Work out the finished part from the listing and answer in its coordinate system (mm). A direction names the side the tool comes from. Give positions to 0.01 mm unless a question says otherwise; leave off trailing zeros. Write each loop counter-clockwise with the first axis right and the second up, starting at its lowest first coordinate (ties: lowest second). Pieces come first, ordered by that corner, then holes.
1) Determine the mould class of faces 1 (the face through (-25, 6, -50)), 2 (the face through (-50, 1, -25)), 3 (the face through (-2.175, 0.789, -46.036)) for opening direction X: pulls with the +X half, pulls with the -X half, needs draft (parallel to the pull), parting line crosses it, or undercut.
2) Find section D-D (z = -28). Determine the outline of the cut face in (x, y), plus the area to 4 significant figures.
3) Find section A-A (z = -47.5). Determine the outline of the cut face in (x, y), plus the area to 3 significant figures.
4) Find section B-B (x = -2.5). Determine the outline of the cut face in (y, z).
5) Given pin 1 Ø5 at (x, y) = (-42, 5.5) entering from +Z; pin 2 Ø4 at (x, z) = (-37.5, -19) entering from +Y; pin 3 Ø3 at (x, y) = (-41.5, 6) entering from -Z, each flat-ended and moving along its own axis, determine where each tip first touches the part or whether it passes through.
6) A tool of negligible diameter and unlimited length cuts with its end or side. For faces 4 (the face through (-3, 7, -10)), 5 (the face through (-43, 5, -45)), 6 (the face through (-8, 7, -25)), 7 (the face through (1, 1.6, -25)), 8 (the face through (-43, 5, -25)), from which of +Z, -Z, +X, -X, +Y, -Y can it reach the whole face along a straight path? Write none if from no direction.
7) Straight lines are drawn through the part: probe 1 along Z at (x, y) = (-47.5, 1); probe 2 along X at (y, z) = (2, -36); probe 3 along X at (y, z) = (10.25, -22.5). For each, find the intervals that lie inside material, in ascending order.
8) Find section C-C (y = 6.25). Determine the outline of the cut face in (x, z), plus the area to 3 significant figures.
Autodesk Inventor part; units mm, degrees
ref_plane "YZ Plane" through (0, 0, 0) normal (1, 0, 0) x (0, 1, 0)
ref_plane "XZ Plane" through (0, 0, 0) normal (0, 1, 0) x (-1, 0, 0)
ref_plane "XY Plane" through (0, 0, 0) normal (0, 0, 1) x (1, 0, 0)
sketch "Sketch1" plane through (0, 0, 0) normal (0, 1, 0) x (-1, 0, 0)
  line L0 (0, 0) -> (50, 0)
  line L1 (50, 0) -> (50, -50)
  line L2 (50, -50) -> (0, -50)
  line L3 (0, -50) -> (0, 0)
  circle A0 centre (47.5, -2.5) radius 1.5
  circle A1 centre (47.5, -47.5) radius 1.5
  circle A2 centre (2.5, -2.5) radius 1.5
  circle A3 centre (2.5, -47.5) radius 1.5
  dimension "d0" = 50
  dimension "d1" = 50
  dimension "d2" = 3
  dimension "d3" = 3
  dimension "d4" = 3
  dimension "d5" = 3
  dimension "d6" = 2.5
  dimension "d7" = 45
  dimension "d8" = 2.5
  dimension "d9" = 2.5
  dimension "d10" = 2.5
  dimension "d11" = 45
  dimension "d12" = 45
  dimension "d13" = 45
extrude "Extrusion1" add sketch "Sketch1" along normal blind 1.6
sketch "Sketch2" plane through (0, 1.6, 0) normal (0, 1, 0) x (1, 0, 0)
  line L0 (-10, 0) -> (-35, 0)
  line L1 (-35, 0) -> (-35, 50)
  line L2 (-35, 50) -> (-10, 50)
  line L3 (-10, 50) -> (-10, 0)
  line L4 (-50, 0) -> (0, 0)
  line L5 (0, 0) -> (0, 50)
  line L6 (2, 10) -> (-8, 10)
  line L7 (-8, 10) -> (-8, 40)
  line L8 (-8, 40) -> (2, 40)
  line L9 (2, 40) -> (2, 10)
  line L10 (-47.5, 45) -> (-38.5, 45)
  line L11 (-38.5, 45) -> (-38.5, 25)
  line L12 (-38.5, 25) -> (-47.5, 25)
  line L13 (-47.5, 25) -> (-47.5, 45)
  line L14 (-50, 50) -> (-50, 0)
  line L15 (0, 50) -> (-50, 50)
  point P0 (0, 40)
  point P1 (0, 10)
  dimension "d16" = 25
  dimension "d17" = 50
  dimension "d19" = 10
  dimension "d20" = 10
  dimension "d21" = 30
  dimension "d22" = 10
  dimension "d23" = 2
  dimension "d26" = 9
  dimension "d27" = 20
  dimension "d28" = 2.5
  dimension "d29" = 5
extrude "Extrusion2" add sketch "Sketch2" along normal blind 10 contours L0 L1 L2 L3 | L6 L7 L8 L5 | L5 L8 L9 L6
extrude "Extrusion3" add sketch "Sketch2" along normal blind 6.5 contours L10 L11 L12 L13
properties part number "motor_driver"
Results:
1. face 1: needs draft
1. face 2: pulls with the -X half
1. face 3: undercut
2. outline: (-50, 0) - (0, 0) - (0, 1.6) - (2, 1.6) - (2, 11.6) - (-8, 11.6) - (-8, 1.6) - (-10, 1.6) - (-10, 11.6) - (-35, 11.6) - (-35, 1.6) - (-38.5, 1.6) - (-38.5, 8.1) - (-47.5, 8.1) - (-47.5, 1.6) - (-50, 1.6) - close
2. area: 488.5 mm2
3. outline: (-50, 0) - (-49, 0) - (-49, 1.6) - (-50, 1.6) - close; (-46, 0) - (-4, 0) - (-4, 1.6) - (-10, 1.6) - (-10, 11.6) - (-35, 11.6) - (-35, 1.6) - (-46, 1.6) - close; (-1, 0) - (0, 0) - (0, 1.6) - (-1, 1.6) - close
3. area: 320 mm2
4. outline: (0, -50) - (1.6, -50) - (1.6, -49) - (0, -49) - close; (0, -46) - (1.6, -46) - (1.6, -40) - (11.6, -40) - (11.6, -10) - (1.6, -10) - (1.6, -4) - (0, -4) - close; (0, -1) - (1.6, -1) - (1.6, 0) - (0, 0) - close
5. pin 1: stops at z = -25
5. pin 2: stops at y = 1.6
5. pin 3: stops at z = -45
6. face 4: +Z, +X, +Y
6. face 5: -Z, -X, +Y
6. face 6: +Z, -Z, +Y
6. face 7: +Z, -Z, +X, -Y
6. face 8: +Z, -X, +Y
7. probe 1: z = -50 to -49, -46 to -4, -1 to 0
7. probe 2: x = -47.5 to -38.5, -35 to -10, -8 to 2
7. probe 3: x = -35 to -10, -8 to 2
8. outline: (-47.5, -45) - (-38.5, -45) - (-38.5, -25) - (-47.5, -25) - close; (-35, -50) - (-10, -50) - (-10, 0) - (-35, 0) - close; (-8, -40) - (2, -40) - (2, -10) - (-8, -10) - close
8. area: 1,730 mm2
